Model file for the job. Use its own axes, mm. Face numbers are marked on the shaded views. Give positions to 0.01 mm unless a question says otherwise; leave off trailing zeros. Write each loop counter-clockwise with the first axis right and the second up, starting at its lowest first coordinate (ties: lowest second). Pieces come first, ordered by that corner, then holes.
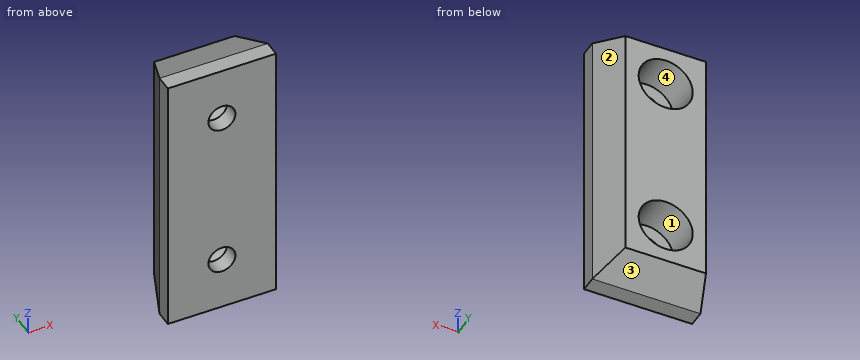
```python
from build123d import *
from OCP.BRepFilletAPI import BRepFilletAPI_MakeChamfer

# Parameters (mm, degrees)
SKETCH1_R             = 5
SKETCH1_R_2           = 2.5
BOSS_EXTRUDE1_DEPTH   = 3
BOSS_EXTRUDE1_2_DEPTH = 3
SKETCH1_3_W           = 20
SKETCH1_3_H           = 50
SKETCH1_3_R           = 5
BOSS_EXTRUDE2_DEPTH   = 10
CHAMFER1_SIZE         = 7
CHAMFER1_SIZE2        = 2.54779164


with BuildPart() as part:
    # Sketch1 → Boss-Extrude1 (new body)
    with BuildSketch(Plane(origin=(0, 0, 0), x_dir=(1, 0, 0), z_dir=(0, 1, 0))):
        with Locations(Location((-10, 40, 0), (0, 0, 270))):
            Circle(SKETCH1_R)
        with Locations(Location((-10, 40, 0), (0, 0, 270))):
            Circle(SKETCH1_R_2, mode=Mode.SUBTRACT)
    extrude(amount=BOSS_EXTRUDE1_DEPTH)



with BuildPart() as body_2:
    # Sketch1 → Boss-Extrude1 2 (new body)
    with BuildSketch(Plane(origin=(0, 0, 0), x_dir=(1, 0, 0), z_dir=(0, 1, 0))):
        with Locations(Location((-10, 10, 0), (0, 0, 270))):
            Circle(SKETCH1_R)
        with Locations(Location((-10, 10, 0), (0, 0, 270))):
            Circle(SKETCH1_R_2, mode=Mode.SUBTRACT)
    extrude(amount=BOSS_EXTRUDE1_2_DEPTH)


with BuildPart() as part_1:
    add(part.part)

    add(body_2.part)  # Boss-Extrude2 merges body 2
    # Sketch1_3 → Boss-Extrude2 (add)
    with BuildSketch(Plane(origin=(0, 0, 0), x_dir=(1, 0, 0), z_dir=(0, 1, 0))):
        with Locations((-10, 25)):
            Rectangle(SKETCH1_3_W, SKETCH1_3_H)
        with Locations(Location((-10, 40, 0), (0, 0, 270))):
            Circle(SKETCH1_3_R, mode=Mode.SUBTRACT)
        with Locations(Location((-10, 10, 0), (0, 0, 270))):
            Circle(SKETCH1_3_R, mode=Mode.SUBTRACT)
    extrude(amount=BOSS_EXTRUDE2_DEPTH)

    # Chamfer1: one chamfer whose edges measure the first distance from different faces: ONE call of the kernel's chamfer builder (chamfer() names one face for all edges)
    chamfer1_edges_1 = [part_1.edges().sort_by_distance(p)[0] for p in [
        (0, 10, -25),
    ]]
    chamfer1_side_1 = [part_1.faces().sort_by_distance(p)[0] for p in [
        (0, 5, -25),
    ]]
    chamfer1_edges_2 = [part_1.edges().sort_by_distance(p)[0] for p in [
        (-10, 10, -50),
    ]]
    chamfer1_side_2 = [part_1.faces().sort_by_distance(p)[0] for p in [
        (-10, 5, -50),
    ]]
    chamfer1_edges_3 = [part_1.edges().sort_by_distance(p)[0] for p in [
        (-20, 10, -25),
    ]]
    chamfer1_side_3 = [part_1.faces().sort_by_distance(p)[0] for p in [
        (-20, 5, -25),
    ]]
    chamfer1_edges_4 = [part_1.edges().sort_by_distance(p)[0] for p in [
        (-10, 10, 0),
    ]]
    chamfer1_side_4 = [part_1.faces().sort_by_distance(p)[0] for p in [
        (-10, 5, 0),
    ]]
    chamfer1 = BRepFilletAPI_MakeChamfer(part_1.part.solid().wrapped)
    for e in chamfer1_edges_1:
        chamfer1.Add(CHAMFER1_SIZE, CHAMFER1_SIZE2, e.wrapped, chamfer1_side_1[0].wrapped)  # the first distance lies on this face
    for e in chamfer1_edges_2:
        chamfer1.Add(CHAMFER1_SIZE, CHAMFER1_SIZE2, e.wrapped, chamfer1_side_2[0].wrapped)  # the first distance lies on this face
    for e in chamfer1_edges_3:
        chamfer1.Add(CHAMFER1_SIZE, CHAMFER1_SIZE2, e.wrapped, chamfer1_side_3[0].wrapped)  # the first distance lies on this face
    for e in chamfer1_edges_4:
        chamfer1.Add(CHAMFER1_SIZE, CHAMFER1_SIZE2, e.wrapped, chamfer1_side_4[0].wrapped)  # the first distance lies on this face
    add(Compound.cast(chamfer1.Shape()), mode=Mode.REPLACE)


solid = part_1.part
```
1. Pin check, flat tips, straight feed: P1, Ø6.5, axis at x = -10, z = -10, coming from the +Y side; P2, Ø6, axis at x = -14.5, y = 7.5, coming from the +Z side; P3, Ø5, axis at y = 8.5, z = -34.5, coming from the -X side. Stop position of each tip, or through.
Calculated:
P1: stops at y = 3
P2: stops at z = -0.55
P3: stops at x = -18.91
2. Slice it at C-C, the plane y = 1. Write the cut outline in (x, z).
Calculated:
outline: (-20, -50) - (0, -50) - (0, 0) - (-20, 0) - close; hole circle Ø5 at (-10, -40); hole circle Ø5 at (-10, -10)
3. Slice it at D-D, the plane z = -31.5. Write the cut outline in (x, y), and give its area (3 significant figures).
Calculated:
outline: (-20, 0) - (0, 0) - (0, 3) - (-2.55, 10) - (-17.45, 10) - (-20, 3) - close
area: 182 mm2
4. Probe probe 1 along Z at (x, y) = (-6.5, 4.75); probe 2 along X at (y, z) = (1.2, -10); probe 3 along Z at (x, y) = (-11.5, 5.5). List the from-to ranges inside material, lowest first.
Calculated:
probe 1: z = -49.36 to -43.57, -36.43 to -13.57, -6.43 to -0.64
probe 2: x = -20 to -12.5, -7.5 to 0
probe 3: z = -49.09 to -44.77, -35.23 to -14.77, -5.23 to -0.91
5. Slice it at B-B, the plane x = -10. Write the cut outline in (y, z), and give its area (3 significant figures).
Calculated:
outline: (0, -50) - (3, -50) - (10, -47.45) - (10, -45) - (3, -45) - (3, -42.5) - (0, -42.5) - close; (0, -37.5) - (3, -37.5) - (3, -35) - (10, -35) - (10, -15) - (3, -15) - (3, -12.5) - (0, -12.5) - close; (0, -7.5) - (3, -7.5) - (3, -5) - (10, -5) - (10, -2.55) - (3, 0) - (0, 0) - close
area: 312 mm2
6. Pull direction Z, two halves, no side cores. Call the marked faces 1, 2, 3 and 4: +Z half, -Z half, draft (parallel to the pull), parting line (faces both ways), or undercut.
Calculated:
face 1: undercut
face 2: draft
face 3: -Z half
face 4: undercut
7. Slice it at A-A, the plane z = -10. Write the cut outline in (x, y).
Calculated:
outline: (-20, 0) - (-12.5, 0) - (-12.5, 3) - (-15, 3) - (-15, 10) - (-17.45, 10) - (-20, 3) - close; (-7.5, 0) - (0, 0) - (0, 3) - (-2.55, 10) - (-5, 10) - (-5, 3) - (-7.5, 3) - close
